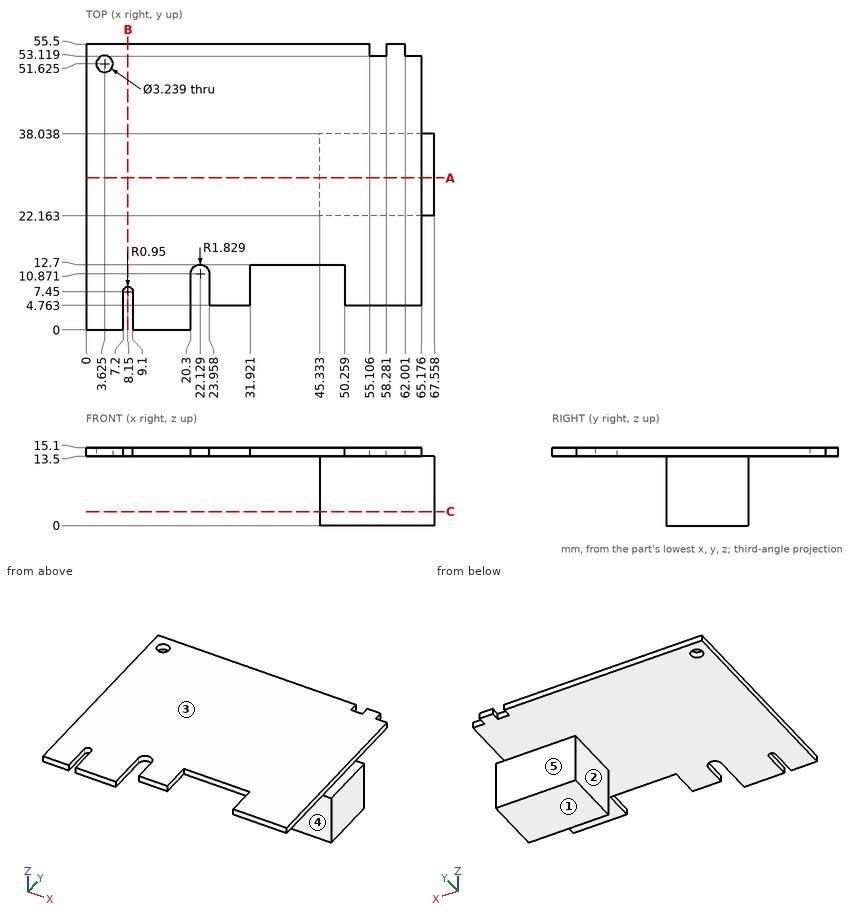
Input: dimensioned drawing with shaded views. Units: mm. Origin: part minimum x, y, z. A direction names the side the tool comes from. Give positions to 0.01 mm unless a question says otherwise; leave off trailing zeros. Write each loop counter-clockwise with the first axis right and the second up, starting at its lowest first coordinate (ties: lowest second). Pieces come first, ordered by that corner, then holes. Notation, with made-up numbers: (31.5, 32.25) - (36.5, 32.25) arc R12 ccw to (36.5, 48.25) - close; hole circle Ø9 at (-6, -21). An arc over 180 degrees is marked (long way). Write item = value, one per line. Start each with the question number.
1) Cut plane C-C (z = 2.75). Return loops of the section in (x, y).
2) Material intervals for L1, parallel to Z at x = 42.5, y = 32; L2, parallel to Y at x = 65, z = 8.5; L3, parallel to X at y = 25.5, z = 6.25, sorted ascending. Write a range as [from, to].
3) Pin query (flat end, axial travel): pin 1 (0.8 mm diameter, centred on x = 56.5, z = 14.5, fed in from -Y); pin 2 (1.8 mm diameter, centred on y = 8, z = 14, fed in from +X); pin 3 (3 mm diameter, centred on x = 33, y = 45, fed in from -Z). Return the tip coordinate at first contact, or that it passes through.
4) Reachability of the marked faces 1, 2, 3, 4 and 5 from +Z, -Z, +X, -X, +Y, -Y: full face, straight path, thin tool, end or side. Return the list, or none.
5) Cut plane A-A (y = 29.5). Return loops of the section in (x, z), and give its area (3 significant figures).
6) Cut plane B-B (x = 8.15). Return loops of the section in (y, z).
Answers follow:
q1.outline = (45.33, 22.16) - (67.56, 22.16) - (67.56, 38.04) - (45.33, 38.04) - close
q2.L1 = [13.5, 15.1]
q2.L2 = [22.16, 38.04]
q2.L3 = [45.33, 67.56]
q3.pin_1 = 4.76
q3.pin_2 = 65.18
q3.pin_3 = 13.5
q4.face_1 = -Z, +X, -X, +Y, -Y
q4.face_2 = -Z, -X, +Y, -Y
q4.face_3 = +Z, +X, -X, +Y, -Y
q4.face_4 = -Z, +X, -X, -Y
q4.face_5 = -Z, +X, -X, +Y
q5.outline = (0, 13.5) - (45.33, 13.5) - (45.33, 0) - (67.56, 0) - (67.56, 13.5) - (65.18, 13.5) - (65.18, 15.1) - (0, 15.1) - close
q5.area = 404 mm^2
q6.outline = (8.4, 13.5) - (55.5, 13.5) - (55.5, 15.1) - (8.4, 15.1) - close
